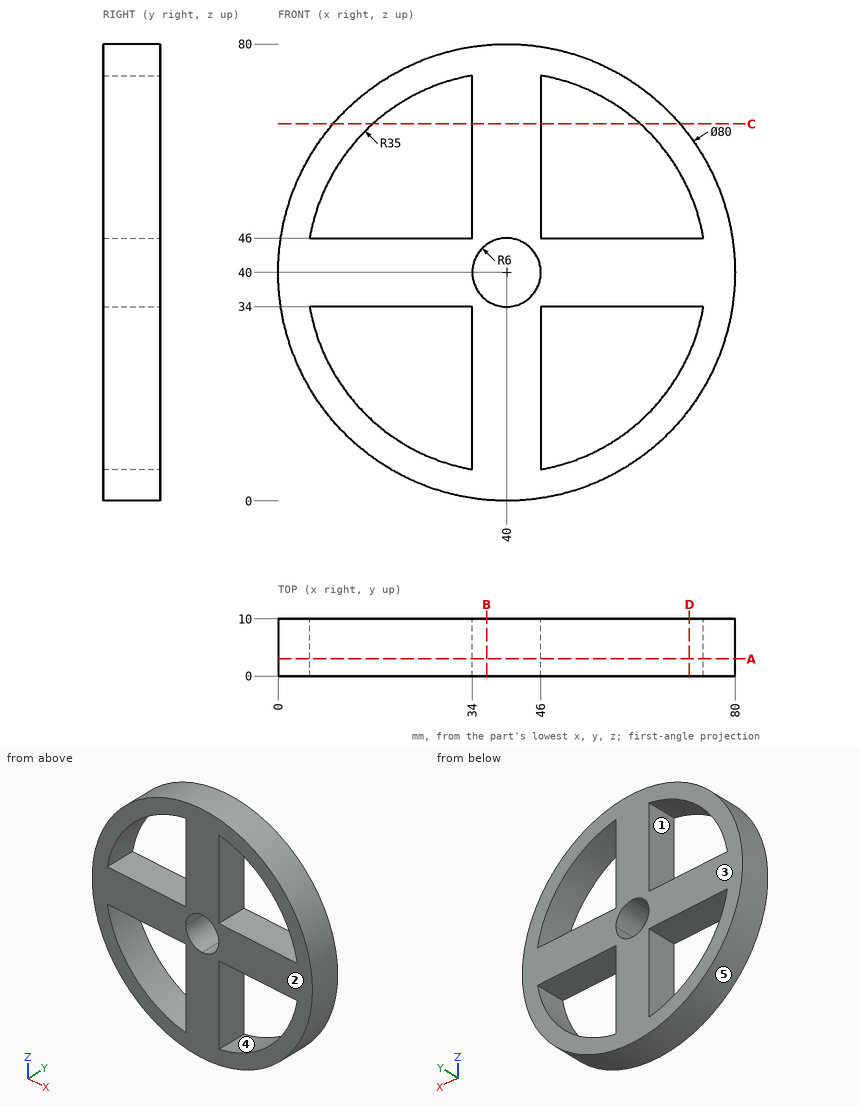
Print and shaded views of the part. All mm, measured from the part's lowest x, y and z. A direction names the side the tool comes from. Give positions to 0.01 mm unless a question says otherwise; leave off trailing zeros. Loops run counter-clockwise (first coordinate to the right, second up) from the corner with the lowest first, then second, coordinate; pieces in that order, holes last. Notation, with made-up numbers: (79.5, -22) - (94.5, -22) arc R21 ccw to (94.5, -1) - close; hole circle Ø5 at (53.5, 50.25). An arc over 180 degrees is marked (long way). One line per item, written item: value. Start each with the question number.
1. Probe L1, parallel to Z at x = 55.5, y = 8.25; L2, parallel to X at y = 7.75, z = 30.5; L3, parallel to X at y = 4.5, z = 14.5. List the from-to ranges inside material, lowest first. Write a range as from..to.
2. Pin check, flat tips, straight feed: pin 1 (5 mm diameter, centred on y = 5.5, z = 22.5, fed in from +X); pin 2 (1 mm diameter, centred on x = 71, y = 5.5, fed in from -Z); pin 3 (5 mm diameter, centred on x = 69, y = 6, fed in from +Z); pin 4 (8 mm diameter, centred on x = 56, z = 51.5, fed in from +Y). Stop position of each tip, or through.
3. Slice it at C-C (z = 66). List the corners of the cut face in (x, y), plus the area to 3 significant figures.
4. Slice it at D-D (x = 72). List the corners of the cut face in (y, z), plus the area to 3 significant figures.
5. Slice it at A-A (y = 3). List the corners of the cut face in (x, z), plus the area to 3 significant figures.
6. Pull direction Z, two halves, no side cores. Call the marked faces 3, 4 and 5: pulls with the +Z half, pulls with the -Z half, needs draft (parallel to the pull), parting line crosses it, or undercut.
7. Slice it at B-B (x = 36.5). List the corners of the cut face in (y, z).
8. Which spindle directions (+Z, -Z, +X, -X, +Y, -Y) get a long thin tool onto all of the face, cutting with end or side? Do the marked faces 1 and 2. Say none if no direction does.
Solution:
1. L1: z = 3.13..8.62, 34..46, 71.38..76.87
1. L2: x = 1.14..6.31, 34..46, 73.69..78.86
1. L3: x = 9.18..16.03, 34..46, 63.97..70.82
2. pin 1: stops at x = 77.08
2. pin 2: stops at z = 14.12
2. pin 3: stops at z = 69.96
2. pin 4: passes through
3. outline: (9.6, 0) - (16.57, 0) - (16.57, 10) - (9.6, 10) - close; (34, 0) - (46, 0) - (46, 10) - (34, 10) - close; (63.43, 0) - (70.4, 0) - (70.4, 10) - (63.43, 10) - close
3. area: 259 mm^2
4. outline: (0, 16) - (10, 16) - (10, 25.82) - (0, 25.82) - close; (0, 34) - (10, 34) - (10, 46) - (0, 46) - close; (0, 54.18) - (10, 54.18) - (10, 64) - (0, 64) - close
4. area: 316 mm^2
5. outline: circle Ø80 at (40, 40); hole (5.52, 34) arc R35 ccw to (34, 5.52) - (34, 34) - close; hole (5.52, 46) - (34, 46) - (34, 74.48) arc R35 ccw to start; hole circle Ø12 at (40, 40); hole (46, 5.52) arc R35 ccw to (74.48, 34) - (46, 34) - close; hole (46, 46) - (74.48, 46) arc R35 ccw to (46, 74.48) - close
5. area: 2,590 mm^2
6. face 3: needs draft
6. face 4: undercut
6. face 5: parting line crosses it
7. outline: (0, 0.15) - (10, 0.15) - (10, 35.13) - (0, 35.13) - close; (0, 44.87) - (10, 44.87) - (10, 79.85) - (0, 79.85) - close
8. face 1: +Y, -Y
8. face 2: +Z, -Z, +X, -X, -Y
